```python
from build123d import *

# Parameters (mm, degrees)
F0_W     = 31.75
F0_H     = 25.4
F1_DEPTH = 6.35
F3_DEPTH = 6.35
F4_W     = 9.525
F4_H     = 6.854803
F5_DEPTH = 6.351


with BuildPart() as f1:
    # F0 (on Front) → F1 (new body)
    with BuildSketch(Plane.XZ):
        with Locations((15.875, 12.7)):
            Rectangle(F0_W, F0_H)
    extrude(amount=F1_DEPTH)

    # F2 (on face) → F3 (cut)
    with BuildSketch(Plane(origin=(0, 0, 0), x_dir=(-1, 0, 0), z_dir=(0, 1, 0))):
        with BuildLine():
            Line((-26.5938, 28.933519), (-26.5938, 25.4))
            ThreePointArc((-26.5938, 25.4), (-15.875, 14.6812), (-5.1562, 25.4))
            Line((-5.1562, 25.4), (-5.135716, 28.933519))
            Line((-5.135716, 28.933519), (-26.5938, 28.933519))
        make_face()
    extrude(amount=-F3_DEPTH, mode=Mode.SUBTRACT)

    # F4 (on face) → F5 (cut, through all)
    with BuildSketch(Plane.XZ.offset(6.35)):
        with Locations((4.7625, 2.414598)):
            Rectangle(F4_W, F4_H)
        with Locations((26.9875, 2.414598)):
            Rectangle(F4_W, F4_H)
    extrude(amount=-F5_DEPTH, mode=Mode.SUBTRACT)


solid = f1.part
```
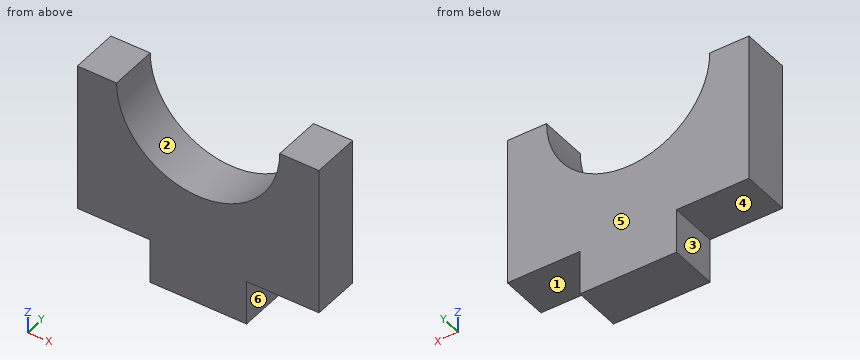
Read the model definition and answer for the solid it produces. Units are mm, in the model's axes. Face numbers are marked on the shaded views. A direction names the side the tool comes from. Round coordinates to 2 decimals unless told otherwise and drop trailing zeros. Write each loop counter-clockwise with the first axis right and the second up, starting at its lowest first coordinate (ties: lowest second). Pieces come first, ordered by that corner, then holes. Notation, with made-up numbers: (-22.75, 47.5) -> (-17.75, 47.5) arc R25 cw to (-17.75, 79.5) -> close; hole circle Ø6 at (44.25, -7). An arc over 180 degrees is marked (long way). Answer in a Markdown table with one row per item. Add a question column.
1) Consider line 1 (X direction, y = -2, z = 18.75); line 2 (Z direction, x = 1, y = -0.25); line 3 (X direction, y = -0.25, z = 18.25). Determine where each line is inside the solid, lowest interval first.
2) Find section A-A, the plane z = 19.25. Determine the outline of the cut face in (x, y), and give its area (3 significant figures).
3) Which of the six approach directions +Z, -Z, +X, -X, +Y, -Y give full straight-line access (tool end or side, diameter ignored) to the marked faces 4, 5 and 6?
4) Find section D-D, the plane z = 22.75. Determine the outline of the cut face in (x, y), and give its area (3 significant figures).
5) Find section B-B, the plane y = -2.25. Determine the outline of the cut face in (x, z) (3 decimals).
6) Find section C-C, the plane x = 25. Determine the outline of the cut face in (y, z), and give its area (3 significant figures).
7) Determine the mould class of the marked faces 1, 2 and 3 for opening direction X: pulls with the +X half, pulls with the -X half, needs draft (parallel to the pull), parting line crosses it, or undercut.
8) Given P1, Ø3, axis at x = 23.5, y = -3.5, coming from the +Z side; P2, Ø3, axis at x = 27, y = -2.5, coming from the -Z side; P3, Ø3, axis at y = -2.5, z = 4, coming from the -X side (3 decimals), each flat-ended and moving along its own axis, determine where each tip first touches the part or whether it passes through.
Findings below:
| question | item | result |
|---|---|---|
| 1 | line 1 | 0 to 7.47, 24.28 to 31.75 |
| 1 | line 2 | 5.84 to 25.4 |
| 1 | line 3 | 0 to 7.89, 23.86 to 31.75 |
| 2 | outline | (0, -6.35) -> (7.1, -6.35) -> (7.1, 0) -> (0, 0) -> close; (24.65, -6.35) -> (31.75, -6.35) -> (31.75, 0) -> (24.65, 0) -> close |
| 2 | area | 90.1 mm² |
| 3 | face 4 | -Z, -X, +Y, -Y |
| 3 | face 5 | +Z, -Z, +X, -X, +Y |
| 3 | face 6 | -Z, +X, +Y, -Y |
| 4 | outline | (0, -6.35) -> (5.49, -6.35) -> (5.49, 0) -> (0, 0) -> close; (26.26, -6.35) -> (31.75, -6.35) -> (31.75, 0) -> (26.26, 0) -> close |
| 4 | area | 69.7 mm² |
| 5 | outline | (0, 5.842) -> (9.525, 5.842) -> (9.525, 0) -> (22.225, 0) -> (22.225, 5.842) -> (31.75, 5.842) -> (31.75, 25.4) -> (26.594, 25.4) arc R10.719 cw to (5.156, 25.4) -> (0, 25.4) -> close |
| 6 | outline | (-6.35, 5.84) -> (0, 5.84) -> (0, 19.78) -> (-6.35, 19.78) -> close |
| 6 | area | 88.5 mm² |
| 7 | face 1 | needs draft |
| 7 | face 2 | undercut |
| 7 | face 3 | pulls with the -X half |
| 8 | P1 | z = 19.78 |
| 8 | P2 | z = 5.84 |
| 8 | P3 | x = 9.525 |
